Solid Edge part; units mm, degrees
sketch "Sketch1" plane through (0, 0, 0) normal (0, -1, 0) x (1, 0, 0)
  line L0 (-39.5, 28) -> (39.5, 28)
  arc A0 (42.5, 25) -> (39.5, 28) centre (39.5, 25) ccw
  line L1 (42.5, 25) -> (42.5, -25)
  arc A1 (39.5, -28) -> (42.5, -25) centre (39.5, -25) ccw
  line L2 (-39.5, -28) -> (39.5, -28)
  arc A2 (-39.5, -28) -> (-42.5, -25) centre (-39.5, -25) cw
  line L3 (-42.5, 25) -> (-42.5, -25)
  arc A3 (-42.5, 25) -> (-39.5, 28) centre (-39.5, 25) cw
  circle A4 centre (19, 24.5) radius 1.375
  circle A5 centre (19, -24.5) radius 1.375
  circle A6 centre (-39, 24.5) radius 1.375
  circle A7 centre (-39, -24.5) radius 1.375
extrude "Protrusion1" add sketch "Sketch1" against normal blind 2
sketch "Sketch2" plane through (0, 0, 0) normal (0, -1, 0) x (1, 0, 0)
  line L0 (45.5, -10.25) -> (23, -10.25)
  line L1 (23, -10.25) -> (23, -25.25)
  line L2 (45.5, -25.25) -> (23, -25.25)
  line L3 (45.5, -10.25) -> (45.5, -25.25)
extrude "RJ45" add sketch "Sketch2" along normal blind 13.5
sketch "Sketch3" plane through (0, 0, 0) normal (0, -1, 0) x (1, 0, 0)
  line L0 (45.5, 24.25) -> (45.5, 13.75)
  line L1 (45.5, 13.75) -> (45.5, 13.25)
  line L2 (45.5, 13.25) -> (45, 13.25)
  line L3 (45, 13.25) -> (45, 13.75)
  line L4 (45, 13.75) -> (25.5, 13.75)
  line L5 (25.5, 13.75) -> (25.5, 24.25)
  line L6 (25.5, 24.25) -> (45, 24.25)
  line L7 (45, 24.75) -> (45, 24.25)
  line L8 (45.5, 24.75) -> (45, 24.75)
  line L9 (45.5, 24.25) -> (45.5, 24.75)
  line L10 (45.5, 6.5) -> (45.5, -4.5)
  line L11 (45.5, -4.5) -> (45.5, -5)
  line L12 (45.5, -5) -> (45, -5)
  line L13 (45, -5) -> (45, -4.5)
  line L14 (25.5, -4.5) -> (45, -4.5)
  line L15 (25.5, 6.5) -> (25.5, -4.5)
  line L16 (45, 6.5) -> (25.5, 6.5)
  line L17 (45, 7) -> (45, 6.5)
  line L18 (45.5, 7) -> (45, 7)
  line L19 (45.5, 6.5) -> (45.5, 7)
extrude "USB" add sketch "Sketch3" along normal blind 16
sketch "Sketch4" plane through (0, 0, 0) normal (0, -1, 0) x (1, 0, 0)
  line L0 (-8.5, 8) -> (-20.5, 8)
  line L1 (-20.5, 8) -> (-20.5, -4)
  line L2 (-20.5, -4) -> (-8.5, -4)
  line L3 (-8.5, -4) -> (-8.5, 8)
extrude "ProtrusiónExtruida_5" add sketch "Sketch4" along normal blind 2.5
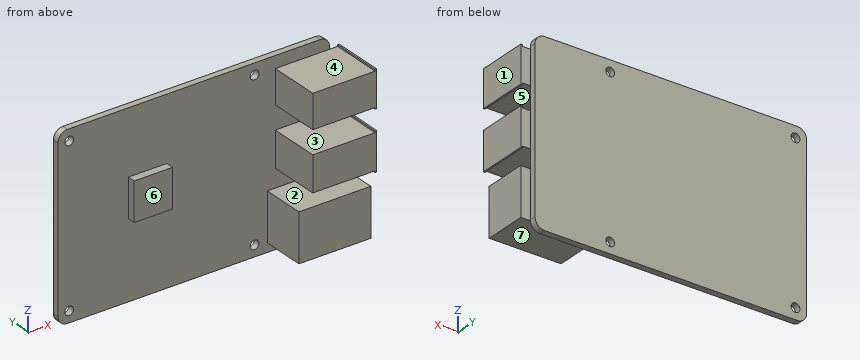
Geometry check sheet. Reference: the model listing, model coordinates, mm. Face numbers are marked on the shaded views. A direction names the side the tool comes from. Give positions to 0.01 mm unless a question says otherwise; leave off trailing zeros. Loops run counter-clockwise (first coordinate to the right, second up) from the corner with the lowest first, then second, coordinate; pieces in that order, holes last.
(1) Thickness scan on L1, parallel to Z at x = 19, y = 1.55 (3 decimals); L2, parallel to Z at x = 26.5, y = -7; L3, parallel to X at y = -0.25, z = -22. Record the ranges inside material, lowest first.
From the geometry:
L1: z = -28 to -25.875, -23.125 to 23.125, 25.875 to 28
L2: z = -25.25 to -10.25, -4.5 to 6.5, 13.75 to 24.25
L3: x = 23 to 45.5
(2) Section check D-D on x = -17. Record the cut outline in (y, z).
From the geometry:
outline: (-2.5, -4) - (0, -4) - (0, -28) - (2, -28) - (2, 28) - (0, 28) - (0, 8) - (-2.5, 8) - close
(3) Section check C-C on z = -18. Record the cut outline in (x, y).
From the geometry:
outline: (-42.5, 0) - (23, 0) - (23, -13.5) - (45.5, -13.5) - (45.5, 0) - (42.5, 0) - (42.5, 2) - (-42.5, 2) - close
(4) Section check B-B on x = 19. Record the cut outline in (y, z) (3 decimals).
From the geometry:
outline: (0, -28) - (2, -28) - (2, -25.875) - (0, -25.875) - close; (0, -23.125) - (2, -23.125) - (2, 23.125) - (0, 23.125) - close; (0, 25.875) - (2, 25.875) - (2, 28) - (0, 28) - close
(5) Set-up check for the marked faces 5, 6 and 7: record each of +Z, -Z, +X, -X, +Y, -Y from which the full face is reachable in a straight line by a thin tool's end or side.
From the geometry:
face 5: -X, -Y
face 6: +Z, -Z, -X, -Y
face 7: -Z, +X, -X, -Y
(6) Depth check by flat-ended pin: pin 1 Ø12 at (x, z) = (10, 10.5) entering from -Y; pin 2 Ø8.5 at (y, z) = (-5, 20.5) entering from -X; pin 3 Ø0.9 at (x, z) = (44.5, -16) entering from +Y. Enter the tip coordinate at first touch or a pass-through.
From the geometry:
pin 1: stops at y = 0
pin 2: stops at x = 25.5
pin 3: stops at y = 0
(7) Release check for a two-part mould opening along Z. For the marked faces 1, 2, 3 and 4 record: released by +Z, released by -Z, zero draft, split by the parting line, or undercut.
From the geometry:
face 1: zero draft
face 2: undercut
face 3: undercut
face 4: released by +Z
(8) Section check A-A on y = -12.5. Record the cut outline in (x, z).
From the geometry:
outline: (23, -25.25) - (45.5, -25.25) - (45.5, -10.25) - (23, -10.25) - close; (25.5, -4.5) - (45, -4.5) - (45, -5) - (45.5, -5) - (45.5, 7) - (45, 7) - (45, 6.5) - (25.5, 6.5) - close; (25.5, 13.75) - (45, 13.75) - (45, 13.25) - (45.5, 13.25) - (45.5, 24.75) - (45, 24.75) - (45, 24.25) - (25.5, 24.25) - close
